Can you work these out from the model? Positions are in its coordinate system, mm. Coordinates: 2 decimals unless noted, no trailing zeros. Order: outer loops, then holes, each group sorted by start corner. A loop starts at its lowest first (then second) coordinate and runs counter-clockwise, first axis right, second up. Notation, with made-up numbers: (86.5, 9) -> (136.5, 9) arc R9 cw to (136.5, 25) -> close; hole circle Ø8 at (35.5, 51). An arc over 180 degrees is marked (long way). Answer as a JSON object with one key per item and string values. Group by question number.
(1) I need wall thicknesses on line 1 (Y direction, x = 3.75, z = -63.5) (3 decimals); line 2 (Z direction, x = 4.25, y = 50.8) (3 decimals); line 3 (Y direction, x = 3.5, z = -38.1) (3 decimals). Which ranges of each line are inside material? Lowest first, please.
(2) I want a section at B-B, the plane z = -43.5. List the corners of the cut face in (x, y) for me.
(3) If we mould it in two halves opening along Y, with no side actions, what happens to faces 1 (the flat face through (0, -7, -57)), 2 (the flat face through (3, -114.3, -35)), 3 (the cylindrical face through (3.13, 28.43, -39.05))? For each: pulls with the +Y half, pulls with the -Y half, needs draft (parallel to the pull), parting line crosses it, or undercut.
(4) I want a section at D-D, the plane x = 3.25. State how many separate pieces and enclosed holes the cut face has, plus the area to 3 significant figures.
(5) I want a section at C-C, the plane z = -12.7. List the corners of the cut face in (x, y) for me (3 decimals), plus the area to 3 significant figures.
(6) For pin 1 (17 mm diameter, centred on y = -31.75, z = -53.975, fed in from -X); pin 2 (1.5 mm diameter, centred on x = 3.5, y = -45, fed in from -Z), each with a flat end and sliding along its axis, tell me the tip position at first contact or that it passes through.
Autodesk Inventor part; units mm, degrees
ref_plane "YZ Plane" through (0, 0, 0) normal (1, 0, 0) x (0, 1, 0)
ref_plane "XZ Plane" through (0, 0, 0) normal (0, 1, 0) x (-1, 0, 0)
ref_plane "XY Plane" through (0, 0, 0) normal (0, 0, 1) x (1, 0, 0)
sketch "Sketch1" plane through (0, 0, 0) normal (1, 0, 0) x (0, 1, 0)
  line L0 (0, 0) -> (63.5, 0)
  line L1 (63.5, 0) -> (63.5, -149.225)
  line L2 (63.5, -149.225) -> (12.7, -149.225)
  circle A0 centre (-31.75, -53.975) radius 14.2875
  line L3 (63.5, -25.4) -> (-43.502, -25.4) construction
  circle A1 centre (50.8, -12.7) radius 3.175
  circle A2 centre (-104.775, -12.7) radius 3.175
  line L4 (12.7, -149.225) -> (-114.3, -69.85)
  line L5 (-114.3, -69.85) -> (-114.3, 0)
  line L6 (-114.3, 0) -> (0, 0)
  circle A3 centre (-85.725, -53.975) radius 14.2875
  line L7 (-53.2384, 0) -> (-95.25, 0)
  circle A4 centre (-79.375, -12.7) radius 3.175
  circle A5 centre (25.4, -38.1) radius 3.175
  circle A6 centre (50.8, -63.5) radius 3.175
  circle A7 centre (22.225, -88.9) radius 3.175
  dimension "d1" = 28.575
  dimension "d2" = 63.5
  dimension "d6" = 25.4
  dimension "d7" = 6.35
  dimension "d8" = 6.35
  dimension "d9" = 12.7
  dimension "d10" = 12.7
  dimension "d12" = 12.7
  dimension "d17" = 50.8
  dimension "d18" = 114.3
  dimension "d19" = 9.525
  dimension "d20" = 53.975
  dimension "d21" = 28.575
  dimension "d24" = 53.975
  dimension "d25" = 69.85
  dimension "d26" = 53.975
  dimension "d27" = 149.225
  dimension "d28" = 107.002
  dimension "d45" = 6.35
  dimension "d46" = 12.7
  dimension "d47" = 25.4
  dimension "d48" = 6.35
  dimension "d49" = 38.1
  dimension "d50" = 38.1
  dimension "d53" = 6.35
  dimension "d54" = 6.35
  dimension "d55" = 41.275
  dimension "d56" = 88.9
  dimension "d57" = 12.7
  dimension "d58" = 63.5
extrude "Extrusion1" add sketch "Sketch1" along normal blind 6.35 contours L0 L1 L2 L4 L5 L6 | A3 | A4 | A5 | A6 | A7
sketch "Sketch2" plane through (0, 0, 0) normal (-1, 0, 0) x (0, 0, 1)
  circle A0 centre (-127, 38.1) radius 14.2875
  line L0 (-149.225, 63.5) -> (-149.225, 12.7)
  line L1 (0, 63.5) -> (-149.225, 63.5)
  point P0 (0, 0)
  dimension "d40" = 28.575
  dimension "d41" = 22.225
  dimension "d42" = 25.4
extrude "Extrusion3" cut sketch "Sketch2" against normal blind 25.4
extrude "Extrusion4" cut sketch "Sketch1" along normal blind 25.4 contours A4 | A5 | A6 | A7
equation "\"BendRadius\" = Thickness"
equation "\"BendReliefWidth\" = Thickness"
equation "\"BendReliefDepth\" = 0.5 * Thickness"
equation "\"CornerReliefSize\" = 4 * Thickness"
equation "\"MinimumRemnant\" = 2 * Thickness"
equation "\"TransitionRadius\" = BendRadius"
equation "\"JacobiRadiusSize\" = Thickness"
equation "\"GapSize\" = Thickness"
properties part number "15102898-16-P-0310" material "Aluminum 6061"
Computed values:
{
 "1": {"line 1": "y = -114.3 to -42.399, -21.101 to 47.625, 53.975 to 63.5", "line 2": "z = -149.225 to -133.545, -120.455 to -66.675, -60.325 to -15.875, -9.525 to 0", "line 3": "y = -114.3 to 22.225, 28.575 to 63.5"},
 "2": {"outline": "(0, -114.3) -> (6.35, -114.3) -> (6.35, -41.47) -> (0, -41.47) -> close; (0, -22.03) -> (6.35, -22.03) -> (6.35, 63.5) -> (0, 63.5) -> close"},
 "3": {"face 1": "needs draft", "face 2": "pulls with the -Y half", "face 3": "undercut"},
 "4": {"separate pieces": "1", "enclosed holes": "8", "area": "20,000 mm2"},
 "5": {"outline": "(0, -114.3) -> (6.35, -114.3) -> (6.35, -107.95) -> (0, -107.95) -> close; (0, -101.6) -> (6.35, -101.6) -> (6.35, -82.55) -> (0, -82.55) -> close; (0, -76.2) -> (6.35, -76.2) -> (6.35, 47.625) -> (0, 47.625) -> close; (0, 53.975) -> (6.35, 53.975) -> (6.35, 63.5) -> (0, 63.5) -> close", "area": "1,010 mm2"},
 "6": {"pin 1": "passes through", "pin 2": "stops at z = -113.63"}
}
